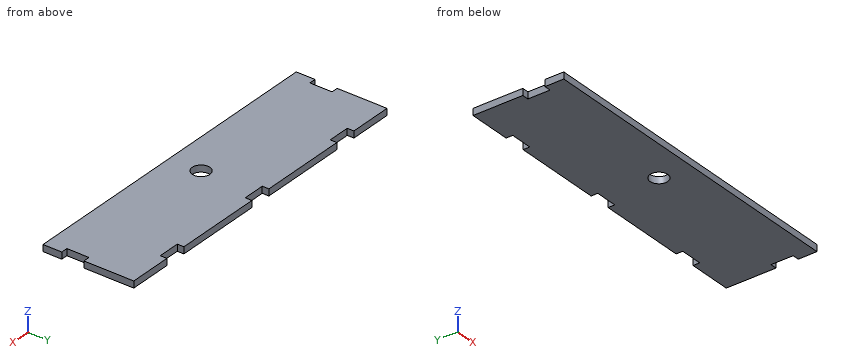
from build123d import *

# Parameters (mm, degrees)
BOSS_EXTRUDE1_DEPTH = 3
SKETCH2_R           = 4
CUT_EXTRUDE1_DEPTH  = 80.298486745


with BuildPart() as part:
    # Sketch1 → Boss-Extrude1 (new body)
    with BuildSketch(Plane.XY):
        Polygon((-74.5, 14), (-74.5, -8.5), (-71.5, -8.5), (-71.5, -18.5), (-74.5, -18.5), (-74.5, -27), (74.5, -27), (74.5, -18.5), (71.5, -18.5), (71.5, -8.5), (74.5, -8.5), (74.5, 14), (55, 14), (55, 11), (45, 11), (45, 14), (5, 14), (5, 11), (-5, 11), (-5, 14), (-45, 14), (-45, 11), (-55, 11), (-55, 14), align=None)
    extrude(amount=BOSS_EXTRUDE1_DEPTH)

    # Sketch2 → Cut-Extrude1 (cut, through all)
    with BuildSketch(Plane.XY):
        with Locations((0, -12.79)):
            Circle(SKETCH2_R)
    extrude(amount=CUT_EXTRUDE1_DEPTH, mode=Mode.SUBTRACT)


solid = part.part
Input: part model. Units: mm. Frame: model coordinates. Coordinates: 2 decimals unless noted, no trailing zeros. Loops run counter-clockwise (first coordinate to the right, second up) from the corner with the lowest first, then second, coordinate; pieces in that order, holes last. Notation, with made-up numbers: (0.5, 36) - (13.5, 36) arc R11 cw to (13.5, 52) - close; hole circle Ø11 at (-37.75, 67.25). An arc over 180 degrees is marked (long way). Answer in a Markdown table with one row per item. Add a question column.
Item 1: Section query A-A on x = 0. Return the cut outline in (y, z), then the cut area to 3 significant figures.
Item 2: Contact query for flat-ended pins moving along their axis: P1, Ø0.9, axis at x = -50.5, z = 1, coming from the +Y side; P2, Ø1, axis at y = -15, z = 1, coming from the +X side; P3, Ø3, axis at x = 14, y = -12, coming from the -Z side. Output: stop coordinate, or through.
Item 3: Section query D-D on x = 52. Return the cut outline in (y, z).
Item 4: Line query: line 1 along X through (y, z) = (12, 2.1); line 2 along X through (y, z) = (-12.79, 1.95); line 3 along Y through (x, z) = (0, 1.3). Output: solid intervals per line, ascending. Write a range as [from, to].
Item 5: Section query B-B on y = -15. Return the cut outline in (x, z).
Item 6: Section query C-C on z = 1.2. Return the cut outline in (x, y).
Recorded:
| question | item | result |
|---|---|---|
| 1 | outline | (-27, 0) - (-16.79, 0) - (-16.79, 3) - (-27, 3) - close; (-8.79, 0) - (11, 0) - (11, 3) - (-8.79, 3) - close |
| 1 | area | 90.0 mm^2 |
| 2 | P1 | y = 11 |
| 2 | P2 | x = 71.5 |
| 2 | P3 | z = 0 |
| 3 | outline | (-27, 0) - (11, 0) - (11, 3) - (-27, 3) - close |
| 4 | line 1 | [-74.5, -55], [-45, -5], [5, 45], [55, 74.5] |
| 4 | line 2 | [-71.5, -4], [4, 71.5] |
| 4 | line 3 | [-27, -16.79], [-8.79, 11] |
| 5 | outline | (-71.5, 0) - (-3.33, 0) - (-3.33, 3) - (-71.5, 3) - close; (3.33, 0) - (71.5, 0) - (71.5, 3) - (3.33, 3) - close |
| 6 | outline | (-74.5, -27) - (74.5, -27) - (74.5, -18.5) - (71.5, -18.5) - (71.5, -8.5) - (74.5, -8.5) - (74.5, 14) - (55, 14) - (55, 11) - (45, 11) - (45, 14) - (5, 14) - (5, 11) - (-5, 11) - (-5, 14) - (-45, 14) - (-45, 11) - (-55, 11) - (-55, 14) - (-74.5, 14) - (-74.5, -8.5) - (-71.5, -8.5) - (-71.5, -18.5) - (-74.5, -18.5) - close; hole circle Ø8 at (0, -12.79) |
